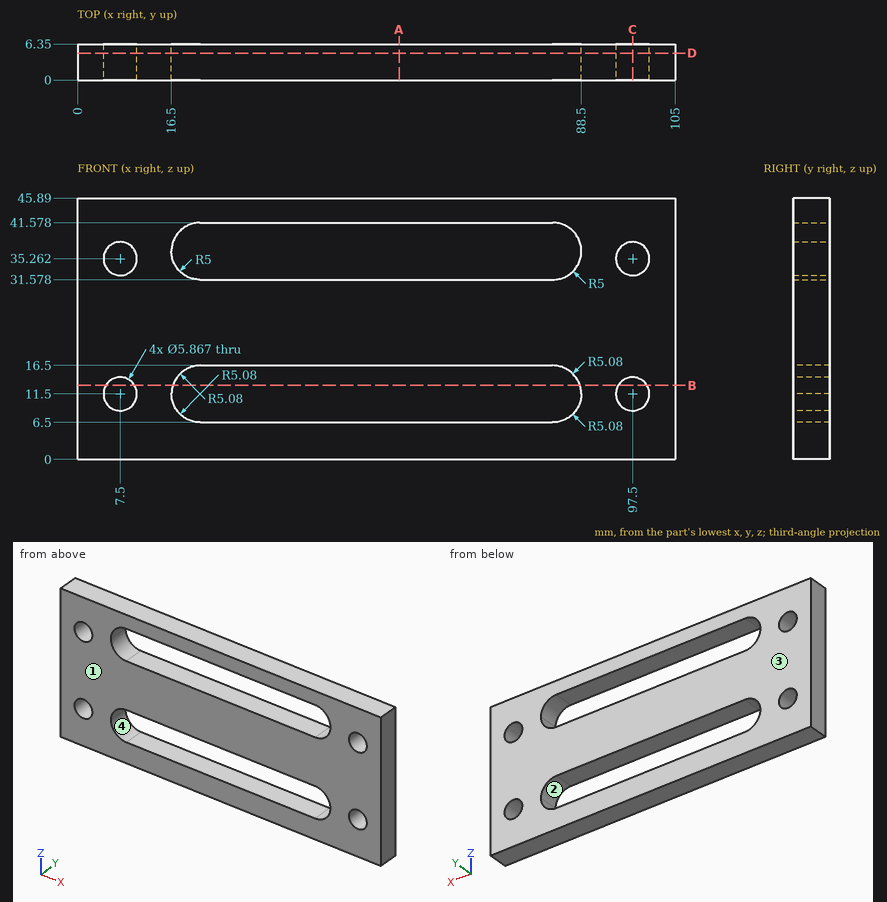
Answer from the drawing. Dimensions are ordinates in mm from the lowest x, y and z of the part. A direction names the side the tool comes from. Round coordinates to 2 decimals unless told otherwise and drop trailing zeros. Order: outer loops, then holes, each group sorted by start corner. A loop starts at its lowest first (then second) coordinate and runs counter-clockwise, first axis right, second up. Notation, with made-up numbers: (28, 64.5) -> (79, 64.5) arc R30 ccw to (79, 94.5) -> close; hole circle Ø11 at (-26, 8.5). An arc over 180 degrees is marked (long way). Answer as CSV lines item,"result".
Q1. For a pull along Z with two mould halves and no side action, classify the marked faces 1 and 2 as +Z half, -Z half, draft (parallel to the pull), parting line (faces both ways), or undercut.
Computed values:
face 1,"draft"
face 2,"undercut"
Q2. A cutting plane is placed at D-D on y = 4.75. Give the number of separate pieces and of enclosed holes in the cut face, plus the area to 3 significant figures.
Computed values:
separate pieces,"1"
enclosed holes,"6"
area,"3,310 mm^2"
Q3. Given pin 1 (5.5 mm diameter, centred on x = 7.5, z = 35.26, fed in from +Y), flat-ended and moving along its own axis, determine where the tip first touches the part or whether it passes through.
Computed values:
pin 1,"passes through"
Q4. A cutting plane is placed at B-B on z = 13. Determine the outline of the cut face in (x, y), plus the area to 3 significant figures.
Computed values:
outline,"(0, 0) -> (4.98, 0) -> (4.98, 6.35) -> (0, 6.35) -> close; (10.02, 0) -> (16.75, 0) -> (16.75, 6.35) -> (10.02, 6.35) -> close; (88.25, 0) -> (94.98, 0) -> (94.98, 6.35) -> (88.25, 6.35) -> close; (100.02, 0) -> (105, 0) -> (105, 6.35) -> (100.02, 6.35) -> close"
area,"149 mm^2"
Q5. Consider line 1 (Z direction, x = 45, y = 0.75); line 2 (Z direction, x = 7.5, y = 3.75); line 3 (X direction, y = 1.75, z = 9) (1 decimal). Determine where each line is inside the solid, lowest interval first. Write a range as from..to.
Computed values:
line 1,"z = 0..6.5, 16.5..31.58, 41.58..45.89"
line 2,"z = 0..8.57, 14.43..32.33, 38.2..45.89"
line 3,"x = 0..6, 9..17.2, 87.8..96, 99..105"
Q6. A cutting plane is placed at C-C on x = 97.5. Determine the outline of the cut face in (y, z), plus the area to 3 significant figures.
Computed values:
outline,"(0, 0) -> (6.35, 0) -> (6.35, 8.57) -> (0, 8.57) -> close; (0, 14.43) -> (6.35, 14.43) -> (6.35, 32.33) -> (0, 32.33) -> close; (0, 38.2) -> (6.35, 38.2) -> (6.35, 45.89) -> (0, 45.89) -> close"
area,"217 mm^2"
Q7. A cutting plane is placed at A-A on x = 56.5. Determine the outline of the cut face in (y, z).
Computed values:
outline,"(0, 0) -> (6.35, 0) -> (6.35, 6.5) -> (0, 6.5) -> close; (0, 16.5) -> (6.35, 16.5) -> (6.35, 31.58) -> (0, 31.58) -> close; (0, 41.58) -> (6.35, 41.58) -> (6.35, 45.89) -> (0, 45.89) -> close"
Q8. Which of the six approach directions +Z, -Z, +X, -X, +Y, -Y give full straight-line access (tool end or side, diameter ignored) to the marked faces 3 and 4?
Computed values:
face 3,"+Z, -Z, +X, -X, +Y"
face 4,"+Y, -Y"
